Check sheet for the modelled part. Datum: model origin and axes. Units: mm. A direction names the side the tool comes from. Give positions to 0.01 mm unless a question says otherwise; leave off trailing zeros. Write each loop counter-clockwise with the first axis right and the second up, starting at its lowest first coordinate (ties: lowest second). Pieces come first, ordered by that corner, then holes. Notation, with made-up numbers: (18, 13) -> (44, 13) arc R18 cw to (44, 32) -> close; hole circle Ø10 at (-5.75, 76). An arc over 180 degrees is marked (long way). Return JSON: item names as keys, results as strings.
from build123d import *

# Parameters (mm, degrees)
BOSS_EXTRUDE1_DEPTH          = 7.5
FILLET1_R                    = 4
M6_CLEARANCE_HOLE1_D         = 6.6
F_4_0_4_DIAMETER_HOLE1_D     = 4
F_4_0_4_DIAMETER_HOLE1_DEPTH = 8
F_4_0_4_DIAMETER_HOLE1_TIP   = 1.201721238
CUT_EXTRUDE1_DEPTH           = 8
CHAMFER1_SIZE                = 3
CUT_EXTRUDE6_DEPTH           = 0.5
CUT_EXTRUDE6_DEPTH_BACK      = 86.255498356
SKETCH12_R                   = 7.525
CUT_EXTRUDE7_DEPTH           = 86.255498356
CUT_EXTRUDE7_DEPTH_BACK      = 86.255498356
SKETCH13_R                   = 6.5
CHAMFER3_SIZE                = 3


with BuildPart() as part:
    # Sketch1 → Boss-Extrude1 (new, symmetric)
    with BuildSketch(Plane.XY):
        Polygon((-11, 0), (11, 0), (11, -70), (28.5, -70), (28.5, -80), (-28.5, -80), (-28.5, -70), (-11, -70), align=None)
    extrude(amount=BOSS_EXTRUDE1_DEPTH, both=True)

    # Fillet1
    fillet1_edges = [part.edges().sort_by_distance(p)[0] for p in [
        (11, -70, 0),
        (-11, -70, 0),
    ]]
    fillet(fillet1_edges, radius=FILLET1_R)

    # M6 Clearance Hole1 (through all)
    with Locations(Plane(origin=(0, -80, 0), x_dir=(-1, 0, 0), z_dir=(0, -1, 0))):
        with Locations((23, 0), (-23, 0)):
            Hole(M6_CLEARANCE_HOLE1_D / 2)

    # Ø4.0 (4) Diameter Hole1
    with Locations(Plane(origin=(0, -80, 0), x_dir=(-1, 0, 0), z_dir=(0, -1, 0))):
        with Locations((12.5, 0)):
            Hole(F_4_0_4_DIAMETER_HOLE1_D / 2, depth=F_4_0_4_DIAMETER_HOLE1_DEPTH)
            with Locations((0, 0, -(F_4_0_4_DIAMETER_HOLE1_DEPTH + F_4_0_4_DIAMETER_HOLE1_TIP / 2))):  # 118° drill point
                Cone(0, F_4_0_4_DIAMETER_HOLE1_D / 2, F_4_0_4_DIAMETER_HOLE1_TIP, mode=Mode.SUBTRACT)

    # Sketch5 → Cut-Extrude1 (cut)
    with BuildSketch(Plane.XZ.offset(80)):
        with BuildLine():
            Line((10, 2), (15, 2))
            ThreePointArc((15, 2), (17, 0), (15, -2))
            Line((15, -2), (10, -2))
            ThreePointArc((10, -2), (8, 0), (10, 2))
        make_face()
    extrude(amount=-CUT_EXTRUDE1_DEPTH, mode=Mode.SUBTRACT)

    # Chamfer1
    chamfer1_edges = [part.edges().sort_by_distance(p)[0] for p in [
        (-28.5, -75, 7.5),
        (28.5, -75, 7.5),
        (28.5, -75, -7.5),
        (-28.5, -75, -7.5),
    ]]
    chamfer(chamfer1_edges, length=CHAMFER1_SIZE)

    # Sketch12 → Cut-Extrude6 (cut, two sides: drawn at the far end of the back side and taken through both)
    with BuildSketch(Plane.XY.offset(-CUT_EXTRUDE6_DEPTH_BACK)):
        with Locations(Location((0, -10, 0), (0, 0, 180))):
            Circle(SKETCH12_R)
    extrude(amount=CUT_EXTRUDE6_DEPTH + CUT_EXTRUDE6_DEPTH_BACK, mode=Mode.SUBTRACT)

    # Sketch13 → Cut-Extrude7 (cut, two sides: drawn at the far end of the back side and taken through both)
    with BuildSketch(Plane.XY.offset(-CUT_EXTRUDE7_DEPTH_BACK)):
        with Locations((0, -10)):
            Circle(SKETCH13_R)
    extrude(amount=CUT_EXTRUDE7_DEPTH + CUT_EXTRUDE7_DEPTH_BACK, mode=Mode.SUBTRACT)

    # Chamfer3
    chamfer3_edges = [part.edges().sort_by_distance(p)[0] for p in [
        (-11, 0, 0),
        (11, 0, 0),
    ]]
    chamfer(chamfer3_edges, length=CHAMFER3_SIZE)


solid = part.part
(1) Release check for a two-part mould opening along X. For faces 6 (the cylindrical face through (-12.203, -68.859, 0.105)), 7 (the flat face through (13, -72, 0)), 8 (the flat face through (0, 0, 0)) record: pulls with the +X half, pulls with the -X half, needs draft (parallel to the pull), parting line crosses it, or undercut.
Reply:
{"face 6": "pulls with the -X half", "face 7": "undercut", "face 8": "needs draft"}
(2) Cross-section at D-D on x = -1.5. Enter the section's corners in (y, z).
Reply:
{"outline": "(-80, -7.5) -> (-17.37, -7.5) -> (-17.37, 0.5) -> (-16.32, 0.5) -> (-16.32, 7.5) -> (-80, 7.5) -> close; (-3.68, 0.5) -> (-2.63, 0.5) -> (-2.63, -7.5) -> (0, -7.5) -> (0, 7.5) -> (-3.68, 7.5) -> close"}
(3) Thickness scan on L1, parallel to Y at x = 0, z = -2 (3 decimals); L2, parallel to X at y = -10, z = 2.25; L3, parallel to Z at x = -23, y = -76.25. Record the ranges inside material, lowest first.
Reply:
{"L1": "-80 to -17.525, -2.475 to 0", "L2": "-11 to -6.5, 6.5 to 11", "L3": "-7.5 to -3.3, 3.3 to 7.5"}
(4) Cross-section at C-C on y = -43.5. Enter the section's corners in (x, z), then the cut area to 3 significant figures.
Reply:
{"outline": "(-11, -7.5) -> (11, -7.5) -> (11, 7.5) -> (-11, 7.5) -> close", "area": "330 mm^2"}
(5) Cross-section at B-B on x = -23. Enter the section's corners in (y, z), then the cut area to 3 significant figures.
Reply:
{"outline": "(-80, -7.5) -> (-70, -7.5) -> (-70, -3.3) -> (-80, -3.3) -> close; (-80, 3.3) -> (-70, 3.3) -> (-70, 7.5) -> (-80, 7.5) -> close", "area": "84.0 mm^2"}
(6) Cross-section at A-A on y = -10. Enter the section's corners in (x, z) (3 decimals).
Reply:
{"outline": "(-11, -7.5) -> (-7.525, -7.5) -> (-7.525, 0.5) -> (-6.5, 0.5) -> (-6.5, 7.5) -> (-11, 7.5) -> close; (6.5, 0.5) -> (7.525, 0.5) -> (7.525, -7.5) -> (11, -7.5) -> (11, 7.5) -> (6.5, 7.5) -> close"}
(7) Set-up check for faces 1 (the flat face through (0, -48, 7.5)), 2 (the flat face through (20, -70, 2)), 3 (the flat face through (0, -48, -7.5)), 4 (the flat face through (13, -76, -2)), 5 (the cylindrical face through (1.631, -2.654, -3.556)): record each of +Z, -Z, +X, -X, +Y, -Y from which the full face is reachable in a straight line by a thin tool's end or side.
Reply:
{"face 1": "+Z, +X, -X, +Y, -Y", "face 2": "+Z, -Z, +X, +Y", "face 3": "-Z, +X, -X, +Y, -Y", "face 4": "-Y", "face 5": "-Z"}
(8) Depth check by flat-ended pin: pin 1 Ø8 at (x, z) = (-17.5, -1) entering from +Y; pin 2 Ø7.5 at (y, z) = (-19.5, -0.5) entering from -X; pin 3 Ø6 at (x, z) = (-23, 0) entering from -Y; pin 4 Ø1.2 at (x, z) = (10.5, 0.5) entering from -Y. Enter the tip coordinate at first touch or a pass-through.
Reply:
{"pin 1": "y = -69.71", "pin 2": "x = -11", "pin 3": "through", "pin 4": "y = -72"}
